```python
from build123d import *

# Parameters (mm, degrees)
SKETCH1_R           = 21.717
SKETCH1_R_2         = 18.542
BOSS_EXTRUDE1_DEPTH = 355.6
CUT_SWEEP1_PITCH    = 203.2
SKETCH17_R          = 21.717
CUT_EXTRUDE3_DEPTH  = 57.15


with BuildPart() as part:
    # Sketch1 → Boss-Extrude1 (new body)
    with BuildSketch(Plane(origin=(0, 0, 0), x_dir=(1, 0, 0), z_dir=(0, 1, 0))):
        with Locations(Location((0, 0, 0), (0, 0, 270))):
            Circle(SKETCH1_R)
        with Locations(Location((0, 0, 0), (0, 0, 270))):
            Circle(SKETCH1_R_2, mode=Mode.SUBTRACT)
    extrude(amount=BOSS_EXTRUDE1_DEPTH)

    # Cut-Sweep1: the profile of Sketch6 profile screwed along a right-hand helix of 0.96 turns, 42 arcs to a turn; built about Z, then put on its axis
    cut_sweep1_z = Axis((0, 0, 0), (0, 0, 1))
    cut_sweep1_corners = [(18.542, 0, -22.86), (21.7173, 0, -22.86), (21.7173, 0, 22.86), (18.542, 0, 22.86)]
    with BuildLine(mode=Mode.PRIVATE) as cut_sweep1_profile:
        Line(cut_sweep1_corners[0], cut_sweep1_corners[1])
        Line(cut_sweep1_corners[1], cut_sweep1_corners[2])
        Line(cut_sweep1_corners[2], cut_sweep1_corners[3])
        Line(cut_sweep1_corners[3], cut_sweep1_corners[0])
    cut_sweep1_cap = Face(cut_sweep1_profile.wire())
    cut_sweep1_turn_angles = [0, 4.285714286, 8.571428571, 12.857142857, 17.142857143, 21.428571429, 25.714285714, 30, 34.285714286, 38.571428571, 42.857142857, 47.142857143, 51.428571429, 55.714285714, 60, 64.285714286, 68.571428571, 72.857142857, 77.142857143, 81.428571429, 85.714285714, 90, 94.285714286, 98.571428571, 102.857142857, 107.142857143, 111.428571429, 115.714285714, 120, 124.285714286, 128.571428571, 132.857142857, 137.142857143, 141.428571429, 145.714285714, 150, 154.285714286, 158.571428571, 162.857142857, 167.142857143, 171.428571429, 175.714285714, 180, 184.285714286, 188.571428571, 192.857142857, 197.142857143, 201.428571429, 205.714285714, 210, 214.285714286, 218.571428571, 222.857142857, 227.142857143, 231.428571429, 235.714285714, 240, 244.285714286, 248.571428571, 252.857142857, 257.142857143, 261.428571429, 265.714285714, 270, 274.285714286, 278.571428571, 282.857142857, 287.142857143, 291.428571429, 295.714285714, 300, 304.285714286, 308.571428571, 312.857142857, 317.142857143, 321.428571429, 325.714285714, 330, 334.285714286, 338.571428571, 342.857142857, 344.228571429, 345.6]
    cut_sweep1_turn_weights = [1, 0.9972037971811801, 1, 0.9972037971811801, 1, 0.9972037971811801, 1, 0.9972037971811801, 1, 0.9972037971811801, 1, 0.9972037971811801, 1, 0.9972037971811801, 1, 0.9972037971811801, 1, 0.9972037971811801, 1, 0.9972037971811801, 1, 0.9972037971811801, 1, 0.9972037971811801, 1, 0.9972037971811801, 1, 0.9972037971811801, 1, 0.9972037971811801, 1, 0.9972037971811801, 1, 0.9972037971811801, 1, 0.9972037971811801, 1, 0.9972037971811801, 1, 0.9972037971811801, 1, 0.9972037971811801, 1, 0.9972037971811801, 1, 0.9972037971811801, 1, 0.9972037971811801, 1, 0.9972037971811801, 1, 0.9972037971811801, 1, 0.9972037971811801, 1, 0.9972037971811801, 1, 0.9972037971811801, 1, 0.9972037971811801, 1, 0.9972037971811801, 1, 0.9972037971811801, 1, 0.9972037971811801, 1, 0.9972037971811801, 1, 0.9972037971811801, 1, 0.9972037971811801, 1, 0.9972037971811801, 1, 0.9972037971811801, 1, 0.9972037971811801, 1, 0.9972037971811801, 1, 0.9997135489685032, 1]
    cut_sweep1_turn_rails = [Edge.make_bspline([Vector(p[0], p[1], 0).rotate(cut_sweep1_z, cut_sweep1_turn_angles[k]) / cut_sweep1_turn_weights[k] + Vector(0, 0, p[2] + CUT_SWEEP1_PITCH * cut_sweep1_turn_angles[k] / 360) for k in range(83)], [0, 0, 0, 1, 1, 2, 2, 3, 3, 4, 4, 5, 5, 6, 6, 7, 7, 8, 8, 9, 9, 10, 10, 11, 11, 12, 12, 13, 13, 14, 14, 15, 15, 16, 16, 17, 17, 18, 18, 19, 19, 20, 20, 21, 21, 22, 22, 23, 23, 24, 24, 25, 25, 26, 26, 27, 27, 28, 28, 29, 29, 30, 30, 31, 31, 32, 32, 33, 33, 34, 34, 35, 35, 36, 36, 37, 37, 38, 38, 39, 39, 40, 40, 41, 41, 41], 2, cut_sweep1_turn_weights) for p in cut_sweep1_corners]
    cut_sweep1_turn_sides = [Face.make_surface_from_curves(cut_sweep1_turn_rails[p[0]], cut_sweep1_turn_rails[p[1]]) for p in [(0, 1), (1, 2), (2, 3), (3, 0)]]
    cut_sweep1 = Plane(origin=(0, 133.35, 0), x_dir=(0, 0, 1), z_dir=(0, 1, 0)) * Solid(Shell([*cut_sweep1_turn_sides, cut_sweep1_cap, cut_sweep1_cap.rotate(cut_sweep1_z, 345.6).moved(Location((0, 0, CUT_SWEEP1_PITCH * 345.6 / 360)))]))
    add(cut_sweep1, mode=Mode.SUBTRACT)

    # Sketch17 → Cut-Extrude3 (cut)
    with BuildSketch(Plane.XZ):
        with Locations(Location((0, 0, 0), (0, 0, 270))):
            Circle(SKETCH17_R)
    extrude(amount=-CUT_EXTRUDE3_DEPTH, mode=Mode.SUBTRACT)


solid = part.part
```
Work out the finished part from the listing and answer in its coordinate system (mm). Coordinates: 2 decimals unless noted, no trailing zeros. Write each loop counter-clockwise with the first axis right and the second up, starting at its lowest first coordinate (ties: lowest second). Pieces come first, ordered by that corner, then holes. Notation, with made-up numbers: (34.5, 46) - (81.5, 46) arc R23 cw to (81.5, 61) - close; hole circle Ø9 at (46.25, 46). An arc over 180 degrees is marked (long way). Answer as a JSON object with one key per item and string values.
Q1. Given pin 1 Ø4 at (y, z) = (305.5, -10) entering from -X; pin 2 Ø6 at (x, y) = (-8.5, 124.5) entering from -Z; pin 3 Ø1.5 at (x, z) = (-10, -13) entering from -Y; pin 4 Ø6 at (x, y) = (1, 286.5) entering from -Z, each flat-ended and moving along its own axis, determine where each tip first touches the part or whether it passes through.
Results list:
{"pin 1": "stops at x = -20.19", "pin 2": "stops at z = -21.01", "pin 3": "passes through", "pin 4": "stops at z = -21.72"}
Q2. For a pull along Z with two mould halves and no side action, classify faces 1 (the cylindrical face through (6.523, 204.286, 20.714)), 2 (the cylindrical face through (0.815, 204.286, -18.524)), 3 (the flat face through (10, 355.6, 16)) as pulls with the +Z half, pulls with the -Z half, needs draft (parallel to the pull), parting line crosses it, or undercut.
Results list:
{"face 1": "parting line crosses it", "face 2": "undercut", "face 3": "needs draft"}
Q3. Consider L1, parallel to Z at x = 0, y = 259; L2, parallel to X at y = 186, z = 0; L3, parallel to Z at x = 2.5, y = 333.5. Determine where each line is inside the solid, lowest interval first. Write a range as from..to.
Results list:
{"L1": "z = -21.72..-18.54, 18.54..21.72", "L2": "x = -21.72..-18.54", "L3": "z = -21.57..-18.37, 18.37..21.57"}
Q4. Find section B-B (x = 9). State how many separate pieces and enclosed holes the cut face has, plus the area to 3 significant figures.
Results list:
{"separate pieces": "4", "enclosed holes": "0", "area": "1,800 mm^2"}
Q5. Find section A-A (y = 79). Write down the section's boundary in (x, z), plus the area to 3 significant figures.
Results list:
{"outline": "circle Ø43.43 at (0, 0); hole circle Ø37.08 at (0, 0)", "area": "402 mm^2"}
